Model file for the job. Use its own axes, mm. Round coordinates to 2 decimals unless told otherwise and drop trailing zeros. Order: outer loops, then holes, each group sorted by start corner. A loop starts at its lowest first (then second) coordinate and runs counter-clockwise, first axis right, second up. Notation, with made-up numbers: (16.5, 30) -> (20.5, 30) arc R26 ccw to (20.5, 44) -> close; hole circle Ø11 at (-12, -28.5). An arc over 180 degrees is marked (long way). Use CSV: the item, a comma, the result in double quotes.
```python
from build123d import *

# Parameters (mm, degrees)
DODANIE_WYCI_GNI_CIE1_START = -9.7
SZKIC2_R                    = 2.1
DODANIE_WYCI_GNI_CIE1_DEPTH = 5


with BuildPart() as part:
    # Szkic2 → Dodanie-wyciągnięcie1 (new body)
    with BuildSketch(Plane(origin=(0, 0, 16.9), x_dir=(-1, 0, 0), z_dir=(0, 0, -1)).offset(DODANIE_WYCI_GNI_CIE1_START)):
        with BuildLine():
            ThreePointArc((-9.222220763, 7.677932287), (0, 12), (9.222220763, 7.677932287))
            Line((9.222220763, 7.677932287), (3.562363692, 21.322711203))
            ThreePointArc((3.562363692, 21.322711203), (0, 23.8), (-3.562363692, 21.322711203))
            Line((-3.562363692, 21.322711203), (-9.222220763, 7.677932287))
        make_face()
        with Locations((0, 20)):
            Circle(SZKIC2_R, mode=Mode.SUBTRACT)
    extrude(amount=-DODANIE_WYCI_GNI_CIE1_DEPTH)


solid = part.part
```
Q1. Cut at D-D (x = -5.75). Give the cut face in (y, z).
From the geometry:
outline,"(10.53, 26.6) -> (16.05, 26.6) -> (16.05, 31.6) -> (10.53, 31.6) -> close"
Q2. Pin check, flat tips, straight feed: pin 1 (2 mm diameter, centred on x = -2, z = 28, fed in from -Y); pin 2 (1 mm diameter, centred on y = 22, z = 28, fed in from +X); pin 3 (2 mm diameter, centred on y = 17, z = 29.5, fed in from +X); pin 4 (5.5 mm diameter, centred on x = 0, y = 20, fed in from -Z). Stop position of each tip, or through.
From the geometry:
pin 1,"stops at y = 11.62"
pin 2,"stops at x = 3.49"
pin 3,"stops at x = 5.77"
pin 4,"stops at z = 26.6"
Q3. Cut at A-A (x = 0). Give the cut face in (y, z), plus the area to 3 significant figures.
From the geometry:
outline,"(12, 26.6) -> (17.9, 26.6) -> (17.9, 31.6) -> (12, 31.6) -> close; (22.1, 26.6) -> (23.8, 26.6) -> (23.8, 31.6) -> (22.1, 31.6) -> close"
area,"38.0 mm²"
Q4. Probe line 1 along X through (y, z) = (21.5, 30.4); line 2 along X through (y, z) = (20.5, 29.5); line 3 along Y through (x, z) = (-1.25, 27.65). List the from-to ranges inside material, lowest first.
From the geometry:
line 1,"x = -3.49 to -1.47, 1.47 to 3.49"
line 2,"x = -3.9 to -2.04, 2.04 to 3.9"
line 3,"y = 11.93 to 18.31, 21.69 to 23.59"
Q5. Mould opens along X. For faces 1 (the flat face through (0, 16, 31.6)), 2 (the flat face through (-6.432, 14.405, 29.065)), 3 (the cylindrical face through (0, 12, 29)), 4 (the flat face through (6.35, 14.6, 29.06)) say: +X half, -X half, draft (parallel to the pull), parting line (faces both ways), or undercut.
From the geometry:
face 1,"draft"
face 2,"-X half"
face 3,"undercut"
face 4,"+X half"
Q6. Cut at B-B (y = 20). Give the cut face in (x, z).
From the geometry:
outline,"(-4.11, 26.6) -> (-2.1, 26.6) -> (-2.1, 31.6) -> (-4.11, 31.6) -> close; (2.1, 26.6) -> (4.11, 26.6) -> (4.11, 31.6) -> (2.1, 31.6) -> close"
Q7. Cut at C-C (z = 29.8). Give the cut face in (x, y), plus the area to 3 significant figures.
From the geometry:
outline,"(-9.22, 7.68) arc R12 cw to (9.22, 7.68) -> (3.56, 21.32) arc R3.8 ccw to (-3.56, 21.32) -> close; hole circle Ø4.2 at (0, 20)"
area,"118 mm²"
